Work out the finished part from the listing and answer in its coordinate system (mm). A direction names the side the tool comes from. Coordinates: 2 decimals unless noted, no trailing zeros. Order: outer loops, then holes, each group sorted by start corner. A loop starts at its lowest first (then second) coordinate and runs counter-clockwise, first axis right, second up. Notation, with made-up numbers: M 26.5,3 L 32.5,3 A31 ccw 32.5,38 Z; hole C 23.25,78.5 d8. An arc over 180 degrees is marked long. Use a Markdown table: item, result.
from build123d import *

# Parameters (mm, degrees)
SKETCH1_W               = 19.8
SKETCH1_H               = 14.4
BOSS_EXTRUDE1_DEPTH     = 14.5
SKETCH3_W               = 7.9
SKETCH3_H               = 14.5
CUT_EXTRUDE1_DEPTH      = 0.8
SKETCH4_W               = 7.9
SKETCH4_H               = 7
CUT_EXTRUDE2_DEPTH      = 23.208556909
MIRROR2_COPY_1_SKETCH_W = 7.9
MIRROR2_COPY_1_SKETCH_H = 14.5
MIRROR2_COPY_1_DEPTH    = 0.8
BOSS_EXTRUDE2_DEPTH     = 7.5
FILLET1_R               = 0.1
CUT_EXTRUDE3_DEPTH      = 7.5
SKETCH7_R               = 1
CUT_EXTRUDE4_DEPTH      = 5
SKETCH8_W               = 2.5
SKETCH8_H               = 1.25
CUT_EXTRUDE5_DEPTH      = 2.5


with BuildPart() as part:
    # Sketch1 → Boss-Extrude1 (new body)
    with BuildSketch(Plane(origin=(0, 0, 0), x_dir=(1, 0, 0), z_dir=(0, 1, 0))):
        Rectangle(SKETCH1_W, SKETCH1_H)
    extrude(amount=BOSS_EXTRUDE1_DEPTH)

    # Sketch3 → Cut-Extrude1 (cut)
    with BuildSketch(Plane.XY.offset(7.2)):
        with Locations((4.95, 7.25)):
            Rectangle(SKETCH3_W, SKETCH3_H)
    cut_extrude1 = extrude(amount=-CUT_EXTRUDE1_DEPTH, mode=Mode.SUBTRACT)

    # Mirror1: Cut-Extrude1 across plane
    add(cut_extrude1.mirror(Plane.XY), mode=Mode.SUBTRACT)

    # Sketch4 → Cut-Extrude2 (cut, through all)
    with BuildSketch(Plane.XY.offset(6.4)):
        with Locations((4.95, 11)):
            Rectangle(SKETCH4_W, SKETCH4_H)
    cut_extrude2 = extrude(amount=-CUT_EXTRUDE2_DEPTH, mode=Mode.SUBTRACT)

    # Mirror2: Cut-Extrude1, Cut-Extrude2 across plane
    add(cut_extrude1.mirror(Plane(origin=(0, 0, 0), x_dir=(0, 0, 1), z_dir=(1, 0, 0))), mode=Mode.SUBTRACT)
    add(cut_extrude2.mirror(Plane(origin=(0, 0, 0), x_dir=(0, 0, 1), z_dir=(1, 0, 0))), mode=Mode.SUBTRACT)

    # Mirror2 copy 1 sketch → Mirror2 copy 1 (cut)
    with BuildSketch(Plane(origin=(0, 0, -7.2), x_dir=(-1, 0, 0), z_dir=(0, 0, -1))):
        with Locations((4.95, 7.25)):
            Rectangle(MIRROR2_COPY_1_SKETCH_W, MIRROR2_COPY_1_SKETCH_H)
    extrude(amount=-MIRROR2_COPY_1_DEPTH, mode=Mode.SUBTRACT)

    # Sketch5 → Boss-Extrude2 (add)
    with BuildSketch(Plane(origin=(0, 7.5, 0), x_dir=(1, 0, 0), z_dir=(0, 1, 0))):
        Polygon((9.9, 5), (9.9, 3.8), (10.8, 3.9), (10.8, 4.9), align=None)
        Polygon((9.9, -5), (9.9, -3.8), (10.8, -3.9), (10.8, -4.9), align=None)
    extrude(amount=-BOSS_EXTRUDE2_DEPTH)

    # Fillet1
    fillet1_edges = [part.edges().sort_by_distance(p)[0] for p in [
        (-8.9, 3.75, 6.4),
        (-1, 3.75, 6.4),
        (8.9, 3.75, 6.4),
        (8.9, 3.75, -6.4),
        (1, 3.75, -6.4),
        (4.95, 7.5, -6.4),
        (1, 3.75, 6.4),
        (1, 7.5, 0),
        (8.9, 7.5, 0),
        (4.95, 7.5, 6.4),
        (-8.9, 3.75, -6.4),
        (-1, 3.75, -6.4),
        (-4.95, 7.5, -6.4),
        (-1, 7.5, 0),
        (-4.95, 7.5, 6.4),
        (-8.9, 7.5, 0),
    ]]
    fillet(fillet1_edges, radius=FILLET1_R)

    # Sketch6 → Cut-Extrude3 (cut)
    with BuildSketch(Plane(origin=(0, 7.5, 0), x_dir=(1, 0, 0), z_dir=(0, 1, 0))):
        Polygon((-9.9, 5.05), (-9.9, 3.75), (-8.9, 3.85), (-8.9, 4.95), align=None)
        Polygon((-9.9, -5.05), (-9.9, -3.75), (-8.9, -3.85), (-8.9, -4.95), align=None)
    extrude(amount=-CUT_EXTRUDE3_DEPTH, mode=Mode.SUBTRACT)

    # Sketch7 → Cut-Extrude4 (cut)
    with BuildSketch(Plane.XZ):
        with Locations(Location((-5, -4.4, 0), (0, 0, 270))):
            Circle(SKETCH7_R)
        with Locations(Location((5, -4.4, 0), (0, 0, 270))):
            Circle(SKETCH7_R)
    extrude(amount=-CUT_EXTRUDE4_DEPTH, mode=Mode.SUBTRACT)

    # Sketch8 → Cut-Extrude5 (cut)
    with BuildSketch(Plane(origin=(0, 7.5, 0), x_dir=(1, 0, 0), z_dir=(0, 1, 0))):
        with Locations((4.95, 4.625)):
            Rectangle(SKETCH8_W, SKETCH8_H)
        with Locations((4.95, -4.625)):
            Rectangle(SKETCH8_W, SKETCH8_H)
    cut_extrude5 = extrude(amount=-CUT_EXTRUDE5_DEPTH, mode=Mode.SUBTRACT)

    # Mirror3: Cut-Extrude5 across plane
    add(cut_extrude5.mirror(Plane(origin=(0, 0, 0), x_dir=(0, 0, 1), z_dir=(1, 0, 0))), mode=Mode.SUBTRACT)


solid = part.part
(1) A cutting plane is placed at B-B (x = -5). Determine the outline of the cut face in (y, z).
Conclusion:
| item | result |
|---|---|
| outline | M 0,-6.4 L 7.4,-6.4 A0.1 ccw 7.5,-6.3 L 7.5,-5.25 L 5,-5.25 L 5,-5.4 L 0,-5.4 Z; M 0,-3.4 L 5,-3.4 L 5,-4 L 7.5,-4 L 7.5,4 L 5,4 L 5,5.25 L 7.5,5.25 L 7.5,6.3 A0.1 ccw 7.4,6.4 L 0,6.4 Z |
(2) Which of the six approach directions +Z, -Z, +X, -X, +Y, -Y give full straight-line access (tool end or side, diameter ignored) to faces 5 (the flat face through (-5, 7.5, 0)), 6 (the flat face through (-6.2, 6, -5)), 7 (the flat face through (-5, 4, -6.4))?
Conclusion:
| item | result |
|---|---|
| face 5 | +Z, -Z, +Y |
| face 6 | +Y |
| face 7 | -Z, +Y, -Y |
(3) A cutting plane is placed at D-D (x = 2.5). Determine the outline of the cut face in (y, z).
Conclusion:
| item | result |
|---|---|
| outline | M 0,-6.4 L 7.4,-6.4 A0.1 ccw 7.5,-6.3 L 7.5,6.3 A0.1 ccw 7.4,6.4 L 0,6.4 Z |
(4) Straight lines are drawn through the part: L1, parallel to X at y = 2.5, z = -4.4; L2, parallel to X at y = 12.25, z = -3.5; L3, parallel to Y at x = -4.75, z = -5.75. For each, find the intervals that lie inside material, in ascending order.
Conclusion:
| item | result |
|---|---|
| L1 | -8.9 to -6, -4 to 4, 6 to 10.8 |
| L2 | -9.9 to -8.9, -1 to 1, 8.9 to 9.9 |
| L3 | 0 to 7.5 |
(5) A cutting plane is placed at A-A (y = 10.5). Determine the outline of the cut face in (x, z).
Conclusion:
| item | result |
|---|---|
| outline | M -9.9,-7.2 L -8.9,-7.2 L -8.9,7.2 L -9.9,7.2 Z; M -1,-7.2 L 1,-7.2 L 1,7.2 L -1,7.2 Z; M 8.9,-7.2 L 9.9,-7.2 L 9.9,7.2 L 8.9,7.2 Z |
(6) Given P1, Ø1.2, axis at x = 4.5, y = 6.5, coming from the +Z side; P2, Ø6, axis at x = 5.5, y = 4, coming from the -Z side; P3, Ø0.6, axis at x = -5, z = 4.5, coming from the +Y side; P4, Ø6, axis at x = -4.5, y = 13, coming from the -Z side, each flat-ended and moving along its own axis, determine where each tip first touches the part or whether it passes through.
Conclusion:
| item | result |
|---|---|
| P1 | z = 6.4 |
| P2 | z = -6.4 |
| P3 | y = 5 |
| P4 | through |
(7) A cutting plane is placed at C-C (z = 0.5). Determine the outline of the cut face in (x, y).
Conclusion:
| item | result |
|---|---|
| outline | M -9.9,0 L 9.9,0 L 9.9,14.5 L 8.9,14.5 L 8.9,7.6 A0.1 cw 8.8,7.5 L 1.1,7.5 A0.1 cw 1,7.6 L 1,14.5 L -1,14.5 L -1,7.6 A0.1 cw -1.1,7.5 L -8.8,7.5 A0.1 cw -8.9,7.6 L -8.9,14.5 L -9.9,14.5 Z |
(8) Determine the mould class of faces 1 (the flat face through (-8.9, 3.8, 4.4)), 2 (the flat face through (10.34, 3.8, 3.85)), 3 (the flat face through (-9.4, 7.1, 7.2)), 4 (the flat face through (-8.9, 10, 0)) for opening direction Z: pulls with the +Z half, pulls with the -Z half, needs draft (parallel to the pull), parting line crosses it, or undercut.
Conclusion:
| item | result |
|---|---|
| face 1 | undercut |
| face 2 | undercut |
| face 3 | pulls with the +Z half |
| face 4 | needs draft |
